For this review, take the finished solid that the model builds, in its own axes (mm). A direction names the side the tool comes from. Coordinates: 2 decimals unless noted, no trailing zeros. Write each loop counter-clockwise with the first axis right and the second up, starting at its lowest first coordinate (ties: lowest second). Pieces come first, ordered by that corner, then holes.
```python
from build123d import *

# Parameters (mm, degrees)
SKETCH_3_W           = 10
SKETCH_3_H           = 35
SKETCH_3_W_2         = 20.75
SKETCH_3_H_2         = 10
SKETCH_3_W_3         = 29.75
SKETCH_3_W_4         = 25
EXTRUDE_1_DEPTH      = 1
EXTRUDE_2_DEPTH      = 4
EXTRUDE_2_DEPTH_BACK = 1
SKETCH_5_W           = 25
SKETCH_5_H           = 10
SKETCH_5_W_2         = 10
SKETCH_5_H_2         = 35
EXTRUDE_3_DEPTH      = 2


with BuildPart() as part:
    # 草图3 → 凸台-拉伸1 (new body)
    with BuildSketch(Plane(origin=(0, 0, 0), x_dir=(1, 0, 0), z_dir=(0, 1, 0))):
        with Locations((17.5, 0)):
            Rectangle(SKETCH_3_W, SKETCH_3_H)
        with Locations((2.125, 0)):
            Rectangle(SKETCH_3_W_2, SKETCH_3_H_2)
        Polygon((-8.25, -5), (-8.25, 5), (-8.25, 20), (-18.25, 20), (-18.25, 5), (-18.25, -5), (-18.25, -20), (-8.25, -20), align=None)
        with Locations((-33.125, 0)):
            Rectangle(SKETCH_3_W_3, SKETCH_3_H_2)
        with Locations((-60.5, 0)):
            Rectangle(SKETCH_3_W_4, SKETCH_3_H_2)
    extrude(amount=EXTRUDE_1_DEPTH)

    # 草图4 → 凸台-拉伸2 (add, two sides)
    with BuildSketch(Plane.XZ) as extrude_2_sk:
        Polygon((11.5, -18.5), (23.5, -18.5), (23.5, 18.5), (11.5, 18.5), (11.5, 6), (-7.25, 6), (-7.25, 21), (-19.25, 21), (-19.25, 6), (-74, 6), (-74, -6), (-19.25, -6), (-19.25, -21), (-7.25, -21), (-7.25, -6), (11.5, -6), align=None)
        Polygon((12.5, -17.5), (22.5, -17.5), (22.5, 17.5), (12.5, 17.5), (12.5, 5), (-8.25, 5), (-8.25, 20), (-18.25, 20), (-18.25, 5), (-73, 5), (-73, -5), (-18.25, -5), (-18.25, -20), (-8.25, -20), (-8.25, -5), (12.5, -5), align=None, mode=Mode.SUBTRACT)
    extrude(amount=EXTRUDE_2_DEPTH)
    extrude(extrude_2_sk.sketch, amount=-EXTRUDE_2_DEPTH_BACK)

    # 草图5 → 凸台-拉伸3 (add)
    with BuildSketch(Plane.XZ):
        Polygon((-18.25, 20), (-18.25, 5), (-14, 5), (-14, -5), (-18.25, -5), (-18.25, -20), (-8.25, -20), (-8.25, -5), (-12.5, -5), (-12.5, 5), (-8.25, 5), (-8.25, 20), align=None)
        with Locations((-60.5, 0)):
            Rectangle(SKETCH_5_W, SKETCH_5_H)
        with Locations((17.5, 0)):
            Rectangle(SKETCH_5_W_2, SKETCH_5_H_2)
    extrude(amount=EXTRUDE_3_DEPTH)


solid = part.part
```
Q1. Add section B-B (z = -0.5). State the section outline as (x, y) points, then the cut area to 4 significant figures.
Ans:
outline: (-74, -4) - (-73, -4) - (-73, -2) - (-48, -2) - (-48, 0) - (-14, 0) - (-14, -2) - (-12.5, -2) - (-12.5, 0) - (12.5, 0) - (12.5, -2) - (22.5, -2) - (22.5, -4) - (23.5, -4) - (23.5, 1) - (-74, 1) - close
area: 178.5 mm2
Q2. Add section D-D (y = -1.2). State the section outline as (x, z) points, then the cut area to 3 significant figures.
Ans:
outline: (-74, -6) - (-19.25, -6) - (-19.25, -21) - (-7.25, -21) - (-7.25, -6) - (11.5, -6) - (11.5, -18.5) - (23.5, -18.5) - (23.5, 18.5) - (11.5, 18.5) - (11.5, 6) - (-7.25, 6) - (-7.25, 21) - (-19.25, 21) - (-19.25, 6) - (-74, 6) - close; hole (-48, -5) - (-14, -5) - (-14, 5) - (-48, 5) - close; hole (-12.5, -5) - (12.5, -5) - (12.5, 5) - (-12.5, 5) - close
area: 1,240 mm2
Q3. Draft analysis for pull direction X (two halves, no side actions). For faces 1 (the flat face through (-74, -2, 0)), 2 (the flat face through (-15, 1, 0)), 3 (the flat face through (17, -2, 0)), state which applies: +X half, -X half, draft (parallel to the pull), parting line (faces both ways), or undercut.
Ans:
face 1: -X half
face 2: draft
face 3: undercut
Q4. Clearance check with flat-ended pins moving along their axes: pin 1 Ø1.5 at (x, y) = (-20.5, -0.5) entering from +Z; pin 2 Ø12 at (x, z) = (-25, -11) entering from -Y; pin 3 Ø2 at (y, z) = (-3.5, -12) entering from -X; pin 4 Ø5 at (x, z) = (17.5, 1) entering from -Y. State where each tip first meets the part, or that it passes through.
Ans:
pin 1: stops at z = 6
pin 2: stops at y = -4
pin 3: stops at x = -19.25
pin 4: stops at y = -2
Q5. Add section A-A (z = -10). State the section outline as (x, y) points.
Ans:
outline: (-19.25, -4) - (-18.25, -4) - (-18.25, -2) - (-8.25, -2) - (-8.25, -4) - (-7.25, -4) - (-7.25, 1) - (-19.25, 1) - close; (11.5, -4) - (12.5, -4) - (12.5, -2) - (22.5, -2) - (22.5, -4) - (23.5, -4) - (23.5, 1) - (11.5, 1) - close
Q6. Tool access review of faces 4 (the flat face through (-18.25, -3, -12)), 5 (the flat face through (11.5, -2, -12)), 6 (the flat face through (-7.25, -2, 13)): name each direction out of +Z, -Z, +X, -X, +Y, -Y from which nothing blocks a thin tool from reaching the whole face with its end or side.
Ans:
face 4: -Y
face 5: -Z, +Y, -Y
face 6: +Z, +Y, -Y
Q7. Add section C-C (x = -44). State the section outline as (y, z) points.
Ans:
outline: (-4, -6) - (1, -6) - (1, 6) - (-4, 6) - (-4, 5) - (0, 5) - (0, -5) - (-4, -5) - close
Q8. For probe 1 along X at (y, z) = (-0.6, 1); probe 2 along X at (y, z) = (-3.35, -16); probe 3 along Z at (x, y) = (-3, -3.15), list the stretches that pass through material, from the lowest coordinate up.
Ans:
probe 1: x = -74 to -48, -14 to -12.5, 12.5 to 23.5
probe 2: x = -19.25 to -18.25, -8.25 to -7.25, 11.5 to 12.5, 22.5 to 23.5
probe 3: z = -6 to -5, 5 to 6
